from build123d import *

# Parameters (mm, degrees)
SKETCH1_R           = 1
BOSS_EXTRUDE1_DEPTH = 1.5
FILLET1_R           = 10
FILLET2_R           = 5
FILLET3_R           = 5
CHAMFER1_SIZE       = 5
FILLET4_R           = 2


with BuildPart() as part:
    # Sketch1 → Boss-Extrude1 (new body)
    with BuildSketch(Plane.XY):
        with BuildLine():
            Line((3.122498999, 2.5), (12.5, 2.5))
            Line((12.5, 2.5), (12.5, 20.5))
            Line((12.5, 20.5), (27.877501001, 20.5))
            ThreePointArc((27.877501001, 20.5), (35, 18), (27.877501001, 15.5))
            Line((27.877501001, 15.5), (17.5, 15.5))
            Line((17.5, 15.5), (17.5, -2.5))
            Line((17.5, -2.5), (3.122498999, -2.5))
            ThreePointArc((3.122498999, -2.5), (-4, 0), (3.122498999, 2.5))
        make_face()
        Circle(SKETCH1_R, mode=Mode.SUBTRACT)
        with Locations((31, 18)):
            Circle(SKETCH1_R, mode=Mode.SUBTRACT)
    extrude(amount=BOSS_EXTRUDE1_DEPTH)

    # Fillet1
    fillet1_edges = [part.edges().sort_by_distance(p)[0] for p in [
        (12.5, 20.5, 0.75),
    ]]
    fillet(fillet1_edges, radius=FILLET1_R)

    # Fillet2
    fillet2_edges = [part.edges().sort_by_distance(p)[0] for p in [
        (17.5, 15.5, 0.75),
    ]]
    fillet(fillet2_edges, radius=FILLET2_R)

    # Fillet3
    fillet3_edges = [part.edges().sort_by_distance(p)[0] for p in [
        (12.5, 2.5, 0.75),
    ]]
    fillet(fillet3_edges, radius=FILLET3_R)

    # Chamfer1
    chamfer1_edges = [part.edges().sort_by_distance(p)[0] for p in [
        (17.5, -2.5, 0.75),
    ]]
    chamfer(chamfer1_edges, length=CHAMFER1_SIZE)

    # Fillet4
    fillet4_edges = [part.edges().sort_by_distance(p)[0] for p in [
        (17.5, 2.5, 0.75),
        (12.5, -2.5, 0.75),
    ]]
    fillet(fillet4_edges, radius=FILLET4_R)


solid = part.part
The model under review builds one solid part; all positions refer to its coordinate system, in mm. A direction names the side the tool comes from. Round coordinates to 2 decimals unless told otherwise and drop trailing zeros. Loops run counter-clockwise (first coordinate to the right, second up) from the corner with the lowest first, then second, coordinate; pieces in that order, holes last. Notation, with made-up numbers: (50, -15.5) -> (75, -15.5) arc R22 ccw to (75, 9.5) -> close; hole circle Ø5 at (82.25, 10.5). An arc over 180 degrees is marked (long way). Return JSON: item names as keys, results as strings.
(1) For faces 1 (the flat face through (25, 20.5, 1)), 2 (the cylindrical face through (19, 14.07, 0.76)), 3 (the flat face through (5, 2.5, 1)), list the 3-axis set-ups (+Z, -Z, +X, -X, +Y, -Y) from which the entire face can be reached by the end or side of a thin tool; tool diameter is ignored.
Solved:
{"face 1": "+Z, -Z, -X, +Y", "face 2": "+Z, -Z, -Y", "face 3": "+Z, -Z, +Y"}
(2) Add section D-D on x = 26. Write out the cut boundary in (y, z).
Solved:
{"outline": "(15.5, 0) -> (20.5, 0) -> (20.5, 1.5) -> (15.5, 1.5) -> close"}
(3) The part is to be moulded in two halves that separate along X. For faces 4 (the cylindrical face through (35, 18, 1)), 5 (the cylindrical face through (17.344, 2.553, 0.76)), 6 (the flat face through (16, 8, 0)), say which applies: released by +X, released by -X, zero draft, split by the parting line, or undercut.
Solved:
{"face 4": "undercut", "face 5": "released by +X", "face 6": "zero draft"}
(4) Add section B-B on y = 18. Write out the cut boundary in (x, z), plus the area to 3 significant figures.
Solved:
{"outline": "(15.89, 0) -> (30, 0) -> (30, 1.5) -> (15.89, 1.5) -> close; (32, 0) -> (35, 0) -> (35, 1.5) -> (32, 1.5) -> close", "area": "25.7 mm2"}
(5) Add section A-A on x = 0. Write out the cut boundary in (y, z).
Solved:
{"outline": "(-4, 0) -> (-1, 0) -> (-1, 1.5) -> (-4, 1.5) -> close; (1, 0) -> (4, 0) -> (4, 1.5) -> (1, 1.5) -> close"}
(6) For line 1 (Y direction, x = 31, z = 0.8); line 2 (Y direction, x = 0, z = 1.25); line 3 (X direction, y = 8.5, z = 0.4), list the stretches that pass through material, from the lowest coordinate up.
Solved:
{"line 1": "14 to 17, 19 to 22", "line 2": "-4 to -1, 1 to 4", "line 3": "12.5 to 17.5"}
(7) Add section C-C on z = 0.6. Write out the cut boundary in (x, y).
Solved:
{"outline": "(3.12, -2.5) -> (11.67, -2.5) arc R2 ccw to (13.09, -1.91) -> (16.91, 1.91) arc R2 ccw to (17.5, 3.33) -> (17.5, 10.5) arc R5 cw to (22.5, 15.5) -> (27.88, 15.5) arc R4 ccw (long way) to (27.88, 20.5) -> (22.5, 20.5) arc R10 ccw to (12.5, 10.5) -> (12.5, 7.5) arc R5 cw to (7.5, 2.5) -> (3.12, 2.5) arc R4 ccw (long way) to start; hole circle Ø2 at (0, 0); hole circle Ø2 at (31, 18)"}
(8) For pin 1 (1.6 mm diameter, centred on x = 31, y = 18, fed in from -Z), flat-tipped, find the tip position at first contact; note if it passes through.
Solved:
{"pin 1": "through"}
